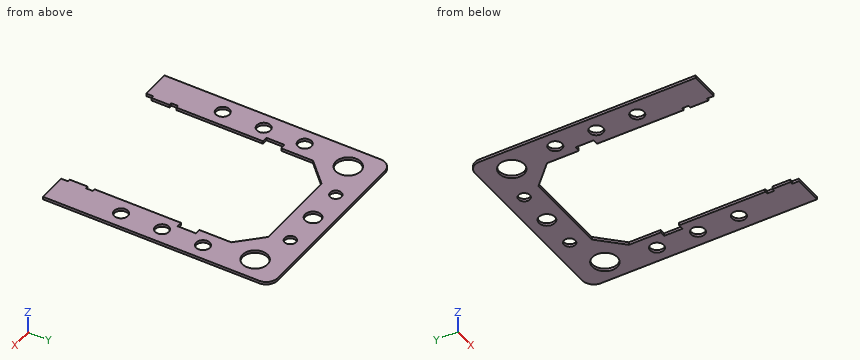
from build123d import *

# Parameters (mm, degrees)
TOWER_DEPTH = 6
SKETCH2_W   = 6
SKETCH2_H   = 15
SKETCH2_W_2 = 12
SKETCH2_H_2 = 40
MOUNT_DEPTH = 615.979674461
FILLET_2_R  = 1
SKETCH3_R   = 12.5
SKETCH3_R_2 = 17.5
SKETCH3_R_3 = 27.5
SKETCH3_R_4 = 15
LITE_DEPTH  = 615.979674461
FILLET2_R   = 25


with BuildPart() as part:
    # Sketch1 → tower (new body)
    with BuildSketch(Plane.XY):
        Polygon((0, 0), (-70, 0), (-70, 500), (358, 500), (358, 0), (288, 0), (288, 370), (238, 420), (50, 420), (0, 370), align=None)
    extrude(amount=-TOWER_DEPTH)

    # Sketch2 → mount (cut, through all)
    with BuildSketch(Plane.XY):
        with Locations((-3, 62.5)):
            Rectangle(SKETCH2_W, SKETCH2_H)
        with Locations((-3, 7.5)):
            Rectangle(SKETCH2_W, SKETCH2_H)
        with Locations((291, 7.5)):
            Rectangle(SKETCH2_W, SKETCH2_H)
        with Locations((291, 62.5)):
            Rectangle(SKETCH2_W, SKETCH2_H)
        with Locations((-6, 280)):
            Rectangle(SKETCH2_W_2, SKETCH2_H_2)
        with Locations((294, 280)):
            Rectangle(SKETCH2_W_2, SKETCH2_H_2)
    extrude(amount=-MOUNT_DEPTH, mode=Mode.SUBTRACT)

    # fillet 2
    fillet_2_edges = [part.edges().sort_by_distance(p)[0] for p in [
        (288, 300, -3),
        (288, 260, -3),
        (-70, 0, -3),
        (358, 0, -3),
        (288, 370, -3),
        (238, 420, -3),
        (50, 420, -3),
        (0, 370, -3),
        (0, 70, -3),
        (-6, 0, -3),
        (288, 70, -3),
        (294, 0, -3),
        (0, 260, -3),
        (0, 300, -3),
    ]]
    fillet(fillet_2_edges, radius=FILLET_2_R)

    # Sketch3 → lite (cut, through all)
    with BuildSketch(Plane.XY):
        with Locations((64, 460)):
            Circle(SKETCH3_R)
        with Locations((144, 460)):
            Circle(SKETCH3_R_2)
        with Locations((224, 460)):
            Circle(SKETCH3_R)
        with Locations((-20, 435)):
            Circle(SKETCH3_R_3)
        with Locations((308, 435)):
            Circle(SKETCH3_R_3)
        with Locations((-35, 330)):
            Circle(SKETCH3_R_4)
        with Locations((-35, 240)):
            Circle(SKETCH3_R_4)
        with Locations((-35, 150)):
            Circle(SKETCH3_R_4)
        with Locations((323, 330)):
            Circle(SKETCH3_R_4)
        with Locations((323, 240)):
            Circle(SKETCH3_R_4)
        with Locations((323, 150)):
            Circle(SKETCH3_R_4)
    extrude(amount=-LITE_DEPTH, mode=Mode.SUBTRACT)

    # fillet2
    fillet2_edges = [part.edges().sort_by_distance(p)[0] for p in [
        (-70, 500, -3),
        (358, 500, -3),
    ]]
    fillet(fillet2_edges, radius=FILLET2_R)


solid = part.part
CAD build for the part. Positions are in the model's coordinates, mm. Give positions to 0.01 mm unless a question says otherwise; leave off trailing zeros. Write each loop counter-clockwise with the first axis right and the second up, starting at its lowest first coordinate (ties: lowest second). Pieces come first, ordered by that corner, then holes. Notation, with made-up numbers: (78.25, -2) -> (128.25, -2) arc R6 cw to (128.25, 2) -> close; hole circle Ø4 at (57.25, 63.5). An arc over 180 degrees is marked (long way). Return JSON: item names as keys, results as strings.
Item 1: Band-saw the part on D-D (x = -35). List the corners of the cut face in (y, z), then the cut area to 3 significant figures.
Answer below:
{"outline": "(0, -6) -> (135, -6) -> (135, 0) -> (0, 0) -> close; (165, -6) -> (225, -6) -> (225, 0) -> (165, 0) -> close; (255, -6) -> (315, -6) -> (315, 0) -> (255, 0) -> close; (345, -6) -> (411.95, -6) -> (411.95, 0) -> (345, 0) -> close; (458.05, -6) -> (500, -6) -> (500, 0) -> (458.05, 0) -> close", "area": "2,180 mm2"}
Item 2: Drop flat-ended pins along their axis: pin 1 (1.5 mm diameter, centred on x = -3.5, z = -4, fed in from -Y); pin 2 (24 mm diameter, centred on x = 323, y = 330, fed in from +Z); pin 3 (1 mm diameter, centred on x = 103, z = -2.5, fed in from -Y). Give the stop position or say it passes through.
Answer below:
{"pin 1": "stops at y = 15", "pin 2": "passes through", "pin 3": "stops at y = 420"}
Item 3: Band-saw the part on B-B (y = 281.5). List the corners of the cut face in (x, z).
Answer below:
{"outline": "(-70, -6) -> (-12, -6) -> (-12, 0) -> (-70, 0) -> close; (300, -6) -> (358, -6) -> (358, 0) -> (300, 0) -> close"}
Item 4: Band-saw the part on C-C (y = 435). List the corners of the cut face in (x, z), then the cut area to 3 significant figures.
Answer below:
{"outline": "(-70, -6) -> (-47.5, -6) -> (-47.5, 0) -> (-70, 0) -> close; (7.5, -6) -> (280.5, -6) -> (280.5, 0) -> (7.5, 0) -> close; (335.5, -6) -> (358, -6) -> (358, 0) -> (335.5, 0) -> close", "area": "1,910 mm2"}
Item 5: Band-saw the part on A-A (x = 224). List the corners of the cut face in (y, z), then the cut area to 3 significant figures.
Answer below:
{"outline": "(420, -6) -> (447.5, -6) -> (447.5, 0) -> (420, 0) -> close; (472.5, -6) -> (500, -6) -> (500, 0) -> (472.5, 0) -> close", "area": "330 mm2"}
Item 6: Drill centre lines: probe 1 along X at (y, z) = (216.5, -3.6); probe 2 along Y at (x, z) = (323, -3.1); probe 3 along X at (y, z) = (452.5, -2.75). Where is each one in solid material? Low to high.
Answer below:
{"probe 1": "x = -70 to 0, 288 to 358", "probe 2": "y = 0 to 135, 165 to 225, 255 to 315, 345 to 411.95, 458.05 to 500", "probe 3": "x = -70 to -41.21, 1.21 to 54, 74 to 128.19, 159.81 to 214, 234 to 286.79, 329.21 to 358"}
